Model file for the job. Use its own axes, mm. A direction names the side the tool comes from. Round coordinates to 2 decimals unless told otherwise and drop trailing zeros. Loops run counter-clockwise (first coordinate to the right, second up) from the corner with the lowest first, then second, coordinate; pieces in that order, holes last. Notation, with made-up numbers: (68, 27) - (91, 27) arc R30 ccw to (91, 50) - close; hole circle Ø11 at (30.5, 26). An arc over 180 degrees is marked (long way). Use one line per item in the form item = value.
from build123d import *

# Parameters (mm, degrees)
F0_W      = 13.5
F0_H      = 26.2
F1_DEPTH  = 2
F2_W      = 18.3
F2_H      = 31
F2_W_2    = 13.5
F2_H_2    = 26.2
F3_DEPTH  = 8.4
F4_R      = 1.5
F5_DEPTH  = 8.4
F6_DEPTH  = 2.4
F7_DEPTH  = 2
F8_DEPTH  = 2
F9_DEPTH  = 1
F10_DEPTH = 0.5
F11_SIZE  = 0.5


with BuildPart() as f1:
    # F0 (on Top) → F1 (new body)
    with BuildSketch(Plane.XY):
        Rectangle(F0_W, F0_H)
        with BuildLine():
            ThreePointArc((2.919408303, 1.1762605042), (0, -10.6), (-2.919408303, 1.1762605042))
            ThreePointArc((-2.919408303, 1.1762605042), (0, 4.55), (2.919408303, 1.1762605042))
        make_face(mode=Mode.SUBTRACT)
    extrude(amount=F1_DEPTH)

    # F2 (on Top) → F3 (join)
    with BuildSketch(Plane.XY):
        Rectangle(F2_W, F2_H)
        Rectangle(F2_W_2, F2_H_2, mode=Mode.SUBTRACT)
    extrude(amount=F3_DEPTH)

    # F4 (on Top) → F5 (join, through all)
    with BuildSketch(Plane.XY):
        with BuildLine():
            Line((-4, 21.1), (-4, 15.5))
            Line((-4, 15.5), (4, 15.5))
            Line((4, 15.5), (4, 21.1))
            ThreePointArc((4, 21.1), (0, 25.1), (-4, 21.1))
        make_face()
        with Locations((0, 21.1)):
            Circle(F4_R, mode=Mode.SUBTRACT)
        with BuildLine():
            Line((4, -21.1), (4, -15.5))
            Line((4, -15.5), (-4, -15.5))
            Line((-4, -15.5), (-4, -21.1))
            ThreePointArc((-4, -21.1), (0, -25.1), (4, -21.1))
        make_face()
        with Locations((0, -21.1)):
            Circle(F4_R, mode=Mode.SUBTRACT)
    extrude(amount=F5_DEPTH)

    # F6 (add): a face of the model
    f6_faces = [f1.faces().sort_by_distance(p)[0] for p in [
        (0, -11.1343154499, 0),
    ]]
    extrude(f6_faces, amount=F6_DEPTH)

    # F7 (cut): a face of the model
    f7_faces = [f1.faces().sort_by_distance(p)[0] for p in [
        (0, -11.1343154499, -2.4),
    ]]
    extrude(f7_faces, amount=-F7_DEPTH, mode=Mode.SUBTRACT)

    # F8 (cut): a face of the model
    f8_faces = [f1.faces().sort_by_distance(p)[0] for p in [
        (0, -11.1343154499, -0.4),
    ]]
    extrude(f8_faces, amount=-F8_DEPTH, mode=Mode.SUBTRACT)

    # F9 (add): a face of the model
    f9_faces = [f1.faces().sort_by_distance(p)[0] for p in [
        (0, -11.1343154499, 1.6),
    ]]
    extrude(f9_faces, amount=F9_DEPTH)

    # F10 (cut): a face of the model
    f10_faces = [f1.faces().sort_by_distance(p)[0] for p in [
        (0, -11.1343154499, 0.6),
    ]]
    extrude(f10_faces, amount=-F10_DEPTH, mode=Mode.SUBTRACT)

    # F11
    f11_edges = [f1.edges().sort_by_distance(p)[0] for p in [
        (0, -10.6, 1.1),
        (0, 4.55, 1.1),
        (9.15, 0, 1.1),
        (6.575, 15.5, 1.1),
        (4, 18.3, 1.1),
        (0, 25.1, 1.1),
        (-4, 18.3, 1.1),
        (-6.575, 15.5, 1.1),
        (-9.15, 0, 1.1),
        (-6.575, -15.5, 1.1),
        (-4, -18.3, 1.1),
        (0, -25.1, 1.1),
        (4, -18.3, 1.1),
        (6.575, -15.5, 1.1),
        (-1.5, 21.1, 1.1),
        (-1.5, -21.1, 1.1),
    ]]
    chamfer(f11_edges, length=F11_SIZE)


solid = f1.part
1. Pull direction X, two halves, no side cores. Call faces 1 (the flat face through (-9.15, 0, 5)), 2 (the flat face through (0, 6, 1.1)), 3 (the cylindrical face through (-0.195, 22.587, 5.048)), 4 (the cylindrical face through (0.232, -10.596, 1.803)): +X half, -X half, draft (parallel to the pull), parting line (faces both ways), or undercut.
Geometry check:
face_1 = -X half
face_2 = draft
face_3 = undercut
face_4 = undercut
2. Tool access for faces 5 (the flat face through (4, 18, 5)), 6 (the flat face through (-7, -15.5, 5)), 7 (the flat face through (-6.75, 0, 5)), 8 (the flat face through (-4, 18, 5)): list every direction of +Z, -Z, +X, -X, +Y, -Y with a clear straight run to the whole face (end or side of a thin tool).
Geometry check:
face_5 = +Z, -Z, +X, +Y
face_6 = +Z, -Z, -X, -Y
face_7 = +Z
face_8 = +Z, -Z, -X, +Y
3. Cut at B-B, the plane z = 4. Give the cut face in (x, y), plus the area to 3 significant figures.
Geometry check:
outline = (-9.15, -15.5) - (-4, -15.5) - (-4, -21.1) arc R4 ccw to (4, -21.1) - (4, -15.5) - (9.15, -15.5) - (9.15, 15.5) - (4, 15.5) - (4, 21.1) arc R4 ccw to (-4, 21.1) - (-4, 15.5) - (-9.15, 15.5) - close; hole (-6.75, -13.1) - (6.75, -13.1) - (6.75, 13.1) - (-6.75, 13.1) - close; hole circle Ø3 at (0, -21.1); hole circle Ø3 at (0, 21.1)
area = 339 mm^2
4. Cut at A-A, the plane y = -4.35. Give the cut face in (x, z).
Geometry check:
outline = (-9.15, 1.6) - (-8.65, 1.1) - (-6.75, 1.1) - (-6.25, 1.6) - (-6.25, 2) - (-6.75, 2) - (-6.75, 8.4) - (-9.15, 8.4) - close; (6.25, 1.6) - (6.75, 1.1) - (8.65, 1.1) - (9.15, 1.6) - (9.15, 8.4) - (6.75, 8.4) - (6.75, 2) - (6.25, 2) - close
5. Cut at C-C, the plane x = -7.25. Give the cut face in (y, z), plus the area to 3 significant figures.
Geometry check:
outline = (-15.5, 1.6) - (-15, 1.1) - (15, 1.1) - (15.5, 1.6) - (15.5, 8.4) - (-15.5, 8.4) - close
area = 226 mm^2
6. Flat gauge pins, fed straight in: pin 1 (1.5 mm diameter, centred on x = 5.5, z = 6.5, fed in from -Y); pin 2 (7.5 mm diameter, centred on x = 0, y = 1.6, fed in from +Z); pin 3 (3 mm diameter, centred on x = -2, z = 4, fed in from -Y). Where does each tip first touch, or does it go through?
Geometry check:
pin_1 = -15.5
pin_2 = 2
pin_3 = -25.07
7. Cut at D-D, the plane y = 11.5. Give the cut face in (x, z), plus the area to 3 significant figures.
Geometry check:
outline = (-9.15, 1.6) - (-8.65, 1.1) - (8.65, 1.1) - (9.15, 1.6) - (9.15, 8.4) - (6.75, 8.4) - (6.75, 2) - (-6.75, 2) - (-6.75, 8.4) - (-9.15, 8.4) - close
area = 46.9 mm^2
8. Wall check: probe 1 along Y at (x, z) = (0, 3.5); probe 2 along X at (y, z) = (-10.5, 4.75); probe 3 along X at (y, z) = (-21, 6). Give the ranges that are in metal, low to high.
Geometry check:
probe_1 = -25.1 to -22.6, -19.6 to -13.1, 13.1 to 19.6, 22.6 to 25.1
probe_2 = -9.15 to -6.75, 6.75 to 9.15
probe_3 = -4 to -1.5, 1.5 to 4
